For this review, use the dimensioned drawing (mm, ordinates from the lowest corner) and the shaded views. A direction names the side the tool comes from. Coordinates: 2 decimals unless noted, no trailing zeros. Write each loop counter-clockwise with the first axis right and the second up, starting at its lowest first coordinate (ties: lowest second). Pieces come first, ordered by that corner, then holes. Notation, with made-up numbers: (39, 63) -> (67, 63) arc R18 cw to (67, 78) -> close; hole circle Ø4 at (9.5, 52.5). An arc over 180 degrees is marked (long way). Put each result on its own line as item: value. Start each with the question number.
Item 1: Insertion check: P1, Ø1, axis at x = 13, z = 7.5, coming from the -Y side; P2, Ø3, axis at x = 5, y = 10, coming from the +Z side; P3, Ø8, axis at y = 10.5, z = 16.5, coming from the +X side. Each pin has a flat end and moves straight along its axis. Give the tip position at first contact, or say it passes through.
Item 2: Consider section C-C on z = 7. Give the boundary of the cut face in (x, y), and give its area (3 significant figures).
Item 3: Consider section A-A on y = 28. Give the boundary of the cut face in (x, z), and give its area (3 significant figures).
Item 4: Consider section D-D on x = 10.75. Give the boundary of the cut face in (y, z).
Item 5: Consider section B-B on x = 7.5. Give the boundary of the cut face in (y, z), and give its area (4 significant figures).
Item 6: To check wall thickness, follow L1, parallel to Z at x = 7.5, y = 21; L2, parallel to Z at x = 7.5, y = 8.5; L3, parallel to X at y = 17, z = 7.25. State the ranges of each line that lie inside material, in increasing order.
Item 7: For the marked faces 1, 2 and 3, list the 3-axis set-ups (+Z, -Z, +X, -X, +Y, -Y) from which the entire face can be reached by the end or side of a thin tool; tool diameter is ignored.
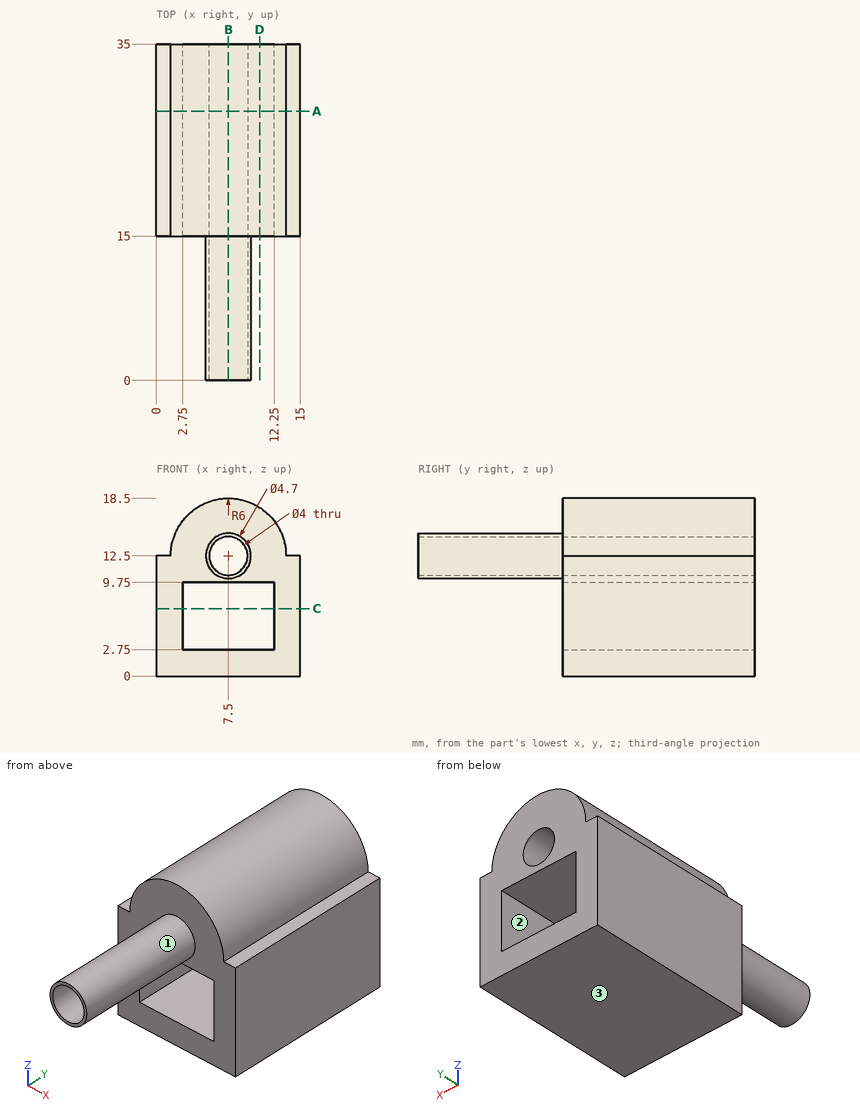
Return value:
1. P1: y = 15
1. P2: z = 14.63
1. P3: x = 9.85
2. outline: (0, 15) -> (2.75, 15) -> (2.75, 35) -> (0, 35) -> close; (12.25, 15) -> (15, 15) -> (15, 35) -> (12.25, 35) -> close
2. area: 110 mm^2
3. outline: (0, 0) -> (15, 0) -> (15, 12.5) -> (13.5, 12.5) arc R6 ccw to (1.5, 12.5) -> (0, 12.5) -> close; hole (2.75, 2.75) -> (12.25, 2.75) -> (12.25, 9.75) -> (2.75, 9.75) -> close; hole circle Ø4 at (7.5, 12.5)
3. area: 165 mm^2
4. outline: (15, 0) -> (35, 0) -> (35, 2.75) -> (15, 2.75) -> close; (15, 9.75) -> (35, 9.75) -> (35, 17.54) -> (15, 17.54) -> close
5. outline: (0, 10.15) -> (15, 10.15) -> (15, 9.75) -> (35, 9.75) -> (35, 10.5) -> (0, 10.5) -> close; (0, 14.5) -> (35, 14.5) -> (35, 18.5) -> (15, 18.5) -> (15, 14.85) -> (0, 14.85) -> close; (15, 0) -> (35, 0) -> (35, 2.75) -> (15, 2.75) -> close
5. area: 160.5 mm^2
6. L1: 0 to 2.75, 9.75 to 10.5, 14.5 to 18.5
6. L2: 10.15 to 10.5, 14.5 to 14.85
6. L3: 0 to 2.75, 12.25 to 15
7. face 1: -Y
7. face 2: +Y, -Y
7. face 3: -Z, +X, -X, +Y, -Y
